Can you work these out from the drawing? Everything is in mm from the part's minimum corner. A direction names the side the tool comes from. Coordinates: 2 decimals unless noted, no trailing zeros. Loops run counter-clockwise (first coordinate to the right, second up) from the corner with the lowest first, then second, coordinate; pieces in that order, holes last. Notation, with made-up numbers: (34.25, -13) - (75.25, -13) arc R36 ccw to (75.25, 26) - close; hole circle Ø4 at (47, 36). An arc over 180 degrees is marked (long way). Use CSV: the item, a comma, the result in double quotes.
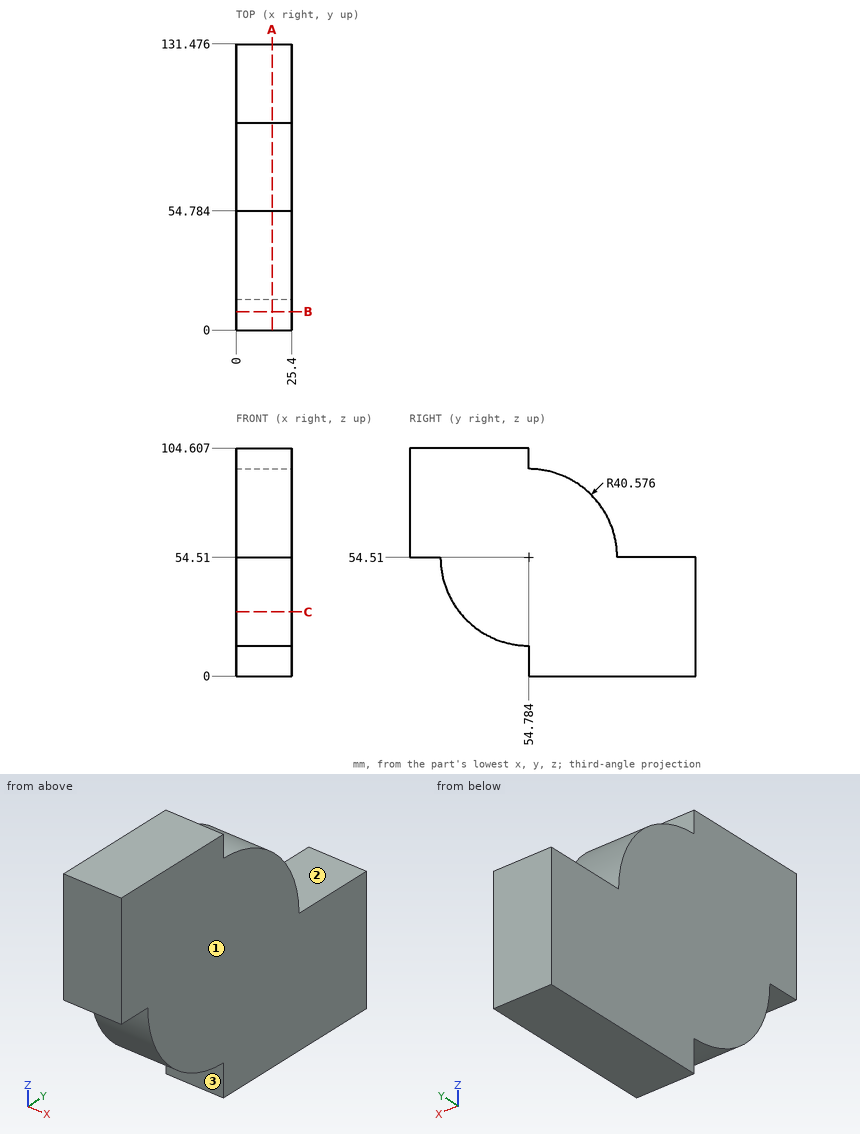
(1) Suppose I cut it at B-B (y = 8.5). Write out the boundary of the cut face in (x, z).
Computed:
outline,"(0, 54.51) - (25.4, 54.51) - (25.4, 104.61) - (0, 104.61) - close"
(2) Suppose I cut it at C-C (z = 29.5). Write out the boundary of the cut face in (x, y) (1 decimal).
Computed:
outline,"(0, 22.8) - (25.4, 22.8) - (25.4, 131.5) - (0, 131.5) - close"
(3) Will these pins go through, and if not, where does the flat tip stop? pin 1 (7 mm diameter, centred on x = 14, y = 10.5, fed in from -Z); pin 2 (7.5 mm diameter, centred on x = 13.5, y = 116.5, fed in from +Z); pin 3 (4 mm diameter, centred on x = 11, z = 80.5, fed in from +Y).
Computed:
pin 1,"stops at z = 54.51"
pin 2,"stops at z = 54.51"
pin 3,"stops at y = 87.51"
(4) Please list where these lines run through material, in increasing order: line 1 (Z direction, x = 14.5, y = 100.5); line 2 (Y direction, x = 14.75, z = 11.5) (1 decimal); line 3 (Z direction, x = 17, y = 11).
Computed:
line 1,"z = 0 to 54.51"
line 2,"y = 54.8 to 131.5"
line 3,"z = 54.51 to 104.61"
(5) Which directions (+Z, -Z, +X, -X, +Y, -Y) give clear straight access to the entire face, cutting with the end or side of a thin tool? Please do the marked faces 1, 2 and 3.
Computed:
face 1,"+Z, -Z, +X, +Y, -Y"
face 2,"+Z, +X, -X, +Y"
face 3,"-Z, +X, -X, -Y"
(6) Suppose I cut it at A-A (x = 16.5). Write out the boundary of the cut face in (y, z) (1 decimal), plus the area to 3 significant figures.
Computed:
outline,"(0, 54.5) - (14.2, 54.5) arc R40.6 ccw to (54.8, 13.9) - (54.8, 0) - (131.5, 0) - (131.5, 54.5) - (95.4, 54.5) arc R40.6 ccw to (54.8, 95.1) - (54.8, 104.6) - (0, 104.6) - close"
area,"9,510 mm²"
